Can you work these out from the model? Positions are in its coordinate system, mm. Face numbers are marked on the shaded views. A direction names the side the tool comes from. Round coordinates to 2 decimals unless told otherwise and drop trailing zeros. Write each loop counter-clockwise with the first axis right and the second up, starting at its lowest first coordinate (ties: lowest second). Pieces come first, ordered by that corner, then holes.
Q1. We'd pull the mould along X, two halves only. Please class the marked faces 1, 2 and 3: +X half, -X half, draft (parallel to the pull), parting line (faces both ways), or undercut.
Q2. If we section it at D-D (y = 0): Please give me the cut outline in (x, z), plus the area to 3 significant figures.
Q3. If we section it at C-C (z = 4.25): Please give me the cut outline in (x, y), plus the area to 3 significant figures.
Q4. If we section it at B-B (x = 21.5): Please give me the cut outline in (y, z).
Q5. I'm going to push flat-ended pins straight in: pin 1 Ø2.5 at (x, z) = (-0.5, 10.5) entering from +Y; pin 2 Ø5.5 at (y, z) = (-16.5, 10) entering from +X; pin 3 Ø3.5 at (x, y) = (21.5, 0) entering from +Z. Where does each tip first touch, or does it pass through?
Q6. If we section it at A-A (y = -11.5): Please give me the cut outline in (x, z), plus the area to 3 significant figures.
Q7. Please list where these lines run through material, in increasing order: line 1 along Y through (x, z) = (2.5, 1.75); line 2 along Y through (x, z) = (4, 6.75); line 3 along Y through (x, z) = (-21.5, 1).
Q8. For the marked faces 4, 5, 6 and 7, which set-ups out of +Z, -Z, +X, -X, +Y, -Y let a thin tool reach every point of the face, with its end or its side?
from build123d import *

# Parameters (mm, degrees)
CROQUIS1_W              = 53
CROQUIS1_H              = 45
CROQUIS1_W_2            = 21.614146676
CROQUIS1_H_2            = 16
CROQUIS1_W_3            = 8.5
CROQUIS1_H_3            = 5.2
SALIENTE_EXTRUIR1_DEPTH = 14.85
CROQUIS2_W              = 9.5
CROQUIS2_H              = 45
CORTAR_EXTRUIR1_DEPTH   = 10
CROQUIS3_W              = 34
CROQUIS3_H              = 17
CORTAR_EXTRUIR2_DEPTH   = 10
CROQUIS4_R              = 1.45
CORTAR_EXTRUIR3_DEPTH   = 10


with BuildPart() as part:
    # Croquis1 → Saliente-Extruir1 (new body)
    with BuildSketch(Plane.XY):
        Rectangle(CROQUIS1_W, CROQUIS1_H)
        with Locations((-0.142926662, -5.5)):
            Rectangle(CROQUIS1_W_2, CROQUIS1_H_2, mode=Mode.SUBTRACT)
        with Locations((0, -17.1)):
            Rectangle(CROQUIS1_W_3, CROQUIS1_H_3, mode=Mode.SUBTRACT)
    extrude(amount=SALIENTE_EXTRUIR1_DEPTH)

    # Croquis2 → Cortar-Extruir1 (cut)
    with BuildSketch(Plane.XY.offset(14.85)):
        with Locations((21.75, 0)):
            Rectangle(CROQUIS2_W, CROQUIS2_H)
        with Locations((-21.75, 0)):
            Rectangle(CROQUIS2_W, CROQUIS2_H)
    extrude(amount=-CORTAR_EXTRUIR1_DEPTH, mode=Mode.SUBTRACT)

    # Croquis3 → Cortar-Extruir2 (cut)
    with BuildSketch(Plane.XY.offset(14.85)):
        with Locations((0, 14)):
            Rectangle(CROQUIS3_W, CROQUIS3_H)
    extrude(amount=-CORTAR_EXTRUIR2_DEPTH, mode=Mode.SUBTRACT)

    # Croquis4 → Cortar-Extruir3 (cut)
    with BuildSketch(Plane.XY.offset(4.85)):
        with Locations((-21.5, 0)):
            Circle(CROQUIS4_R)
        with Locations((21.5, 0)):
            Circle(CROQUIS4_R)
    extrude(amount=-CORTAR_EXTRUIR3_DEPTH, mode=Mode.SUBTRACT)


solid = part.part
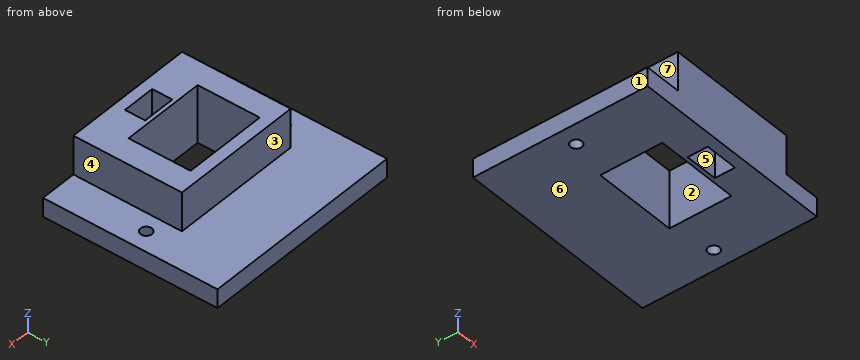
A:
1. face 1: -X half
1. face 2: undercut
1. face 3: draft
2. outline: (-26.5, 0) - (-22.95, 0) - (-22.95, 4.85) - (-26.5, 4.85) - close; (-20.05, 0) - (-10.95, 0) - (-10.95, 14.85) - (-17, 14.85) - (-17, 4.85) - (-20.05, 4.85) - close; (10.66, 0) - (20.05, 0) - (20.05, 4.85) - (17, 4.85) - (17, 14.85) - (10.66, 14.85) - close; (22.95, 0) - (26.5, 0) - (26.5, 4.85) - (22.95, 4.85) - close
2. area: 248 mm2
3. outline: (-26.5, -22.5) - (26.5, -22.5) - (26.5, 22.5) - (-26.5, 22.5) - close; hole circle Ø2.9 at (-21.5, 0); hole (-10.95, -13.5) - (10.66, -13.5) - (10.66, 2.5) - (-10.95, 2.5) - close; hole (-4.25, -19.7) - (4.25, -19.7) - (4.25, -14.5) - (-4.25, -14.5) - close; hole circle Ø2.9 at (21.5, 0)
3. area: 1,980 mm2
4. outline: (-22.5, 0) - (-1.45, 0) - (-1.45, 4.85) - (-22.5, 4.85) - close; (1.45, 0) - (22.5, 0) - (22.5, 4.85) - (1.45, 4.85) - close
5. pin 1: stops at y = 5.5
5. pin 2: stops at x = 17
5. pin 3: stops at z = 4.85
6. outline: (-26.5, 0) - (-10.95, 0) - (-10.95, 14.85) - (-17, 14.85) - (-17, 4.85) - (-26.5, 4.85) - close; (10.66, 0) - (26.5, 0) - (26.5, 4.85) - (17, 4.85) - (17, 14.85) - (10.66, 14.85) - close
6. area: 276 mm2
7. line 1: y = -22.5 to -19.7, -14.5 to -13.5, 2.5 to 22.5
7. line 2: y = -22.5 to -19.7, -14.5 to -13.5, 2.5 to 5.5
7. line 3: y = -22.5 to -1.45, 1.45 to 22.5
8. face 4: +Z, +X, +Y, -Y
8. face 5: +Z, -Z
8. face 6: -Z, +X, -X, +Y, -Y
8. face 7: +Z, -X, +Y, -Y
